Read the model definition and answer for the solid it produces. Units are mm, in the model's axes. A direction names the side the tool comes from. Give positions to 0.01 mm unless a question says otherwise; leave off trailing zeros. Loops run counter-clockwise (first coordinate to the right, second up) from the corner with the lowest first, then second, coordinate; pieces in that order, holes last. Notation, with made-up numbers: (45.25, -20) - (75.25, -20) arc R9 ccw to (75.25, -15) - close; hole circle Ø9 at (-8.5, -20.5). An arc over 180 degrees is marked (long way). Put each result on its own line as item: value. Start each with the question number.
1. A cutting plane is placed at C-C, the plane y = 11. Determine the outline of the cut face in (x, z).
2. Given pin 1 Ø5 at (x, z) = (-8, 3.5) entering from -Y; pin 2 Ø3 at (x, z) = (21.5, 2.5) entering from -Y; pin 3 Ø6 at (y, z) = (10.5, 4.5) entering from -X, each flat-ended and moving along its own axis, determine where each tip first touches the part or whether it passes through.
3. A cutting plane is placed at D-D, the plane z = 0.5. Determine the outline of the cut face in (x, y).
4. A cutting plane is placed at B-B, the plane x = 22.25. Determine the outline of the cut face in (y, z), plus the area to 3 significant figures.
5. A cutting plane is placed at A-A, the plane x = 4. Determine the outline of the cut face in (y, z).
6. Consider L1, parallel to Y at x = 18.5, z = 2.5; L2, parallel to Y at x = 1, z = 2.25; L3, parallel to Y at x = -10.5, z = 8. Determine where each line is inside the solid, lowest interval first. Write a range as from..to.
7. For a pull along Z with two mould halves and no side action, classify faces 5 (the cylindrical face through (-8.75, 23.52, 5.07)), 6 (the flat face through (6, 14, 0)), 7 (the flat face through (20, 4, 5)), 8 (the flat face through (6, 14, 10)) as released by +Z, released by -Z, zero draft, split by the parting line, or undercut.
8. For faces 1 (the flat face through (-4.5, 19, 5)), 2 (the flat face through (15, 23, 5)), 3 (the cylindrical face through (11.75, 23.52, 5.07)), 4 (the flat face through (8.5, 22, 4.9)), determine the directions among +Z, -Z, +X, -X, +Y, -Y from which every point of the face is accessible in a straight line to the end or side of a thin tool.
```python
from build123d import *

# Parameters (mm, degrees)
F0_W     = 9
F0_H     = 1.5
F1_DEPTH = 10
F3_R     = 1.5
F4_DEPTH = 3
F5_DEPTH = 41.751


with BuildPart() as f1:
    # F0 (on Top) → F1 (new body)
    with BuildSketch(Plane.XY):
        Polygon((4.5, 23.5), (4.5, 22), (15, 22), (15, 25), (-15, 25), (-15, 22), (-4.5, 22), (-4.5, 23.5), align=None)
        with Locations((0, 22.75)):
            Rectangle(F0_W, F0_H)
        with BuildLine():
            ThreePointArc((-4.5, 16.1342028003), (0, 16.75), (4.5, 16.1342028003))
            Line((4.5, 16.1342028003), (4.5, 22))
            Line((4.5, 22), (-4.5, 22))
            Line((-4.5, 22), (-4.5, 16.1342028003))
        make_face()
        with BuildLine():
            ThreePointArc((-4.5, 12.9927864602), (0, 13.75), (4.5, 12.9927864602))
            Line((4.5, 12.9927864602), (4.5, 16.1342028003))
            ThreePointArc((4.5, 16.1342028003), (0, 16.75), (-4.5, 16.1342028003))
            Line((-4.5, 16.1342028003), (-4.5, 12.9927864602))
        make_face()
        with BuildLine():
            ThreePointArc((4.5, 12.9927864602), (9.9068234991, 9.5350588964), (13.1553221169, 4))
            Line((13.1553221169, 4), (16.2653773396, 4))
            ThreePointArc((16.2653773396, 4), (12.0253874538, 11.6598694927), (4.5, 16.1342028003))
            Line((4.5, 16.1342028003), (4.5, 12.9927864602))
        make_face()
        with BuildLine():
            ThreePointArc((-13.1553221169, 4), (-9.9068234991, 9.5350588964), (-4.5, 12.9927864602))
            Line((-4.5, 12.9927864602), (-4.5, 16.1342028003))
            ThreePointArc((-4.5, 16.1342028003), (-12.0253874538, 11.6598694927), (-16.2653773396, 4))
            Line((-16.2653773396, 4), (-13.1553221169, 4))
        make_face()
        with BuildLine():
            ThreePointArc((13.1553221169, 4), (13.5179356693, 2.5155347824), (13.7135881519, 1))
            Line((13.7135881519, 1), (16.7201226072, 1))
            ThreePointArc((16.7201226072, 1), (16.5608212866, 2.5103183692), (16.2653773396, 4))
            Line((16.2653773396, 4), (13.1553221169, 4))
        make_face()
        with BuildLine():
            ThreePointArc((16.2653773396, 4), (16.5608212866, 2.5103183692), (16.7201226072, 1))
            Line((16.7201226072, 1), (25, 1))
            Line((25, 1), (25, 4))
            Line((25, 4), (16.2653773396, 4))
        make_face()
        with BuildLine():
            Line((25, -1), (16.7201226072, -1))
            ThreePointArc((16.7201226072, -1), (16.5608212866, -2.5103183692), (16.2653773396, -4))
            Line((16.2653773396, -4), (25, -4))
            Line((25, -4), (25, -1))
        make_face()
        with BuildLine():
            Line((16.7201226072, -1), (13.7135881519, -1))
            ThreePointArc((13.7135881519, -1), (13.5179356693, -2.5155347824), (13.1553221169, -4))
            Line((13.1553221169, -4), (16.2653773396, -4))
            ThreePointArc((16.2653773396, -4), (16.5608212866, -2.5103183692), (16.7201226072, -1))
        make_face()
        with BuildLine():
            Line((16.2653773396, -4), (13.1553221169, -4))
            ThreePointArc((13.1553221169, -4), (9.9068234991, -9.5350588964), (4.5, -12.9927864602))
            Line((4.5, -12.9927864602), (4.5, -16.1342028003))
            ThreePointArc((4.5, -16.1342028003), (12.0253874538, -11.6598694927), (16.2653773396, -4))
        make_face()
        with BuildLine():
            Line((-4.5, -16.1342028003), (-4.5, -12.9927864602))
            ThreePointArc((-4.5, -12.9927864602), (-9.9068234991, -9.5350588964), (-13.1553221169, -4))
            Line((-13.1553221169, -4), (-16.2653773396, -4))
            ThreePointArc((-16.2653773396, -4), (-12.0253874538, -11.6598694927), (-4.5, -16.1342028003))
        make_face()
        with BuildLine():
            ThreePointArc((-13.1553221169, -4), (-13.5179356693, -2.5155347824), (-13.7135881519, -1))
            Line((-13.7135881519, -1), (-16.7201226072, -1))
            ThreePointArc((-16.7201226072, -1), (-16.5608212866, -2.5103183692), (-16.2653773396, -4))
            Line((-16.2653773396, -4), (-13.1553221169, -4))
        make_face()
        with BuildLine():
            ThreePointArc((-13.7135881519, -1), (-13.75, 0), (-13.7135881519, 1))
            Line((-13.7135881519, 1), (-16.7201226072, 1))
            ThreePointArc((-16.7201226072, 1), (-16.75, 0), (-16.7201226072, -1))
            Line((-16.7201226072, -1), (-13.7135881519, -1))
        make_face()
        with BuildLine():
            Line((-16.7201226072, 1), (-13.7135881519, 1))
            ThreePointArc((-13.7135881519, 1), (-13.5179356693, 2.5155347824), (-13.1553221169, 4))
            Line((-13.1553221169, 4), (-16.2653773396, 4))
            ThreePointArc((-16.2653773396, 4), (-16.5608212866, 2.5103183692), (-16.7201226072, 1))
        make_face()
        with BuildLine():
            Line((4.5, -16.1342028003), (4.5, -12.9927864602))
            ThreePointArc((4.5, -12.9927864602), (0, -13.75), (-4.5, -12.9927864602))
            Line((-4.5, -12.9927864602), (-4.5, -16.1342028003))
            ThreePointArc((-4.5, -16.1342028003), (0, -16.75), (4.5, -16.1342028003))
        make_face()
    extrude(amount=F1_DEPTH)

    # F3 (on offset) → F4 (cut, through all)
    with BuildSketch(Plane(origin=(0, 25, 0), x_dir=(-1, 0, 0), z_dir=(0, 1, 0))):
        with Locations((-10.25, 5)):
            Circle(F3_R)
        with Locations((10.25, 5)):
            Circle(F3_R)
        with Locations((-22.25, 5)):
            Circle(F3_R)
    extrude(amount=-F4_DEPTH, mode=Mode.SUBTRACT)

    # F3 (on offset) → F5 (cut, through all)
    with BuildSketch(Plane(origin=(0, 25, 0), x_dir=(-1, 0, 0), z_dir=(0, 1, 0))):
        with Locations((-22.25, 5)):
            Circle(F3_R)
    extrude(amount=-F5_DEPTH, mode=Mode.SUBTRACT)


solid = f1.part
```
Return value:
1. outline: (-12.63, 0) - (-8.25, 0) - (-8.25, 10) - (-12.63, 10) - close; (8.25, 0) - (12.63, 0) - (12.63, 10) - (8.25, 10) - close
2. pin 1: stops at y = -15.82
2. pin 2: stops at y = -4
2. pin 3: stops at x = -14.98
3. outline: (-15, 22) - (-4.5, 22) - (-4.5, 16.13) arc R16.75 ccw (long way) to (16.27, -4) - (25, -4) - (25, -1) - (13.71, -1) arc R13.75 cw (long way) to (13.71, 1) - (25, 1) - (25, 4) - (16.27, 4) arc R16.75 ccw to (4.5, 16.13) - (4.5, 22) - (15, 22) - (15, 25) - (-15, 25) - close
4. outline: (-4, 0) - (-1, 0) - (-1, 3.5) - (-4, 3.5) - close; (-4, 6.5) - (-1, 6.5) - (-1, 10) - (-4, 10) - close; (1, 0) - (4, 0) - (4, 3.5) - (1, 3.5) - close; (1, 6.5) - (4, 6.5) - (4, 10) - (1, 10) - close
4. area: 42.0 mm2
5. outline: (-16.27, 0) - (-13.16, 0) - (-13.16, 10) - (-16.27, 10) - close; (13.16, 0) - (25, 0) - (25, 10) - (13.16, 10) - close
6. L1: y = -4..-1, 1..4
6. L2: y = -16.72..-13.71, 13.71..25
6. L3: y = -13.05..-8.88, 8.88..13.05, 22..25
7. face 5: undercut
7. face 6: released by -Z
7. face 7: zero draft
7. face 8: released by +Z
8. face 1: +Z, -Z, -X
8. face 2: +Z, -Z, +X, +Y
8. face 3: +Y
8. face 4: +Z, -Z, +X
